Read the model definition and answer for the solid it produces. Units are mm, in the model's axes. A direction names the side the tool comes from. Give positions to 0.01 mm unless a question says otherwise; leave off trailing zeros. Write each loop counter-clockwise with the first axis right and the second up, starting at its lowest first coordinate (ties: lowest second). Pieces come first, ordered by that corner, then holes. Notation, with made-up numbers: M -14,43 L 45,43 A19 ccw 45,48 Z; hole C 12.5,14.5 d8. An arc over 180 degrees is marked long. Put each result on its own line as item: value.
from build123d import *

# Parameters (mm, degrees)
SKETCH1_R           = 12.7
EXTRUDE1_DEPTH      = 11.1125
EXTRUDE2_DEPTH      = 23.225
SKETCH4_R           = 2.3876
BOSS_EXTRUDE1_DEPTH = 19.05


with BuildPart() as part:
    # Sketch1 → Extrude1 (new body, symmetric)
    with BuildSketch(Plane.XY):
        Circle(SKETCH1_R)
    extrude(amount=EXTRUDE1_DEPTH, both=True)

    # Sketch2 → Extrude2 (cut, through all)
    with BuildSketch(Plane.XY.offset(11.1125)):
        with BuildLine():
            ThreePointArc((0.79375, 2.24506403), (0, 2.38125), (-0.79375, 2.24506403))
            Line((-0.79375, 2.24506403), (-0.79375, 1.5875))
            Line((-0.79375, 1.5875), (0.79375, 1.5875))
            Line((0.79375, 1.5875), (0.79375, 2.24506403))
        make_face()
        with BuildLine():
            Line((-0.79375, 1.5875), (-0.79375, 2.24506403))
            ThreePointArc((-0.79375, 2.24506403), (-1.374815329, -1.944282483), (2.38125, 0))
            ThreePointArc((2.38125, 0), (1.944282483, 1.374815329), (0.79375, 2.24506403))
            Line((0.79375, 2.24506403), (0.79375, 1.5875))
            Line((0.79375, 1.5875), (-0.79375, 1.5875))
        make_face()
        with BuildLine():
            Line((0.79375, 3.175), (-0.79375, 3.175))
            Line((-0.79375, 3.175), (-0.79375, 2.24506403))
            ThreePointArc((-0.79375, 2.24506403), (0, 2.38125), (0.79375, 2.24506403))
            Line((0.79375, 2.24506403), (0.79375, 3.175))
        make_face()
    extrude(amount=-EXTRUDE2_DEPTH, mode=Mode.SUBTRACT)

    # Sketch4 → Boss-Extrude1 (add, symmetric)
    with BuildSketch(Plane.XY):
        Circle(SKETCH4_R)
    extrude(amount=BOSS_EXTRUDE1_DEPTH, both=True)


solid = part.part
(1) Section B-B on z = -1 is taken. Determine the outline of the cut face in (x, y) (3 decimals).
Result:
outline: C 0,0 d25.4; hole M -0.794,2.252 A2.388 cw 0.794,2.252 L 0.794,3.175 L -0.794,3.175 Z
(2) Straight lines are drawn through the part: line 1 along Z through (x, y) = (-1.25, -9); line 2 along Y through (x, z) = (-0.5, 2) (3 decimals); line 3 along X through (y, z) = (-9.75, -5). For each, find the intervals that lie inside material, in ascending order. Write a range as from..to.
Result:
line 1: z = -11.11..11.11
line 2: y = -12.69..2.335, 3.175..12.69
line 3: x = -8.14..8.14
(3) For a pull along Y with two mould halves and no side action, classify faces 4 (the face through (0, -3, -11.112)), 5 (the face through (0.794, 3, 0)), 6 (the face through (-2.75, -12.4, 0.16)) as +Y half, -Y half, draft (parallel to the pull), parting line (faces both ways), or undercut.
Result:
face 4: draft
face 5: undercut
face 6: parting line
(4) Section C-C on y = 0 is taken. Determine the outline of the cut face in (x, z), and give its area (3 significant figures).
Result:
outline: M -12.7,-11.11 L -2.39,-11.11 L -2.39,-19.05 L 2.39,-19.05 L 2.39,-11.11 L 12.7,-11.11 L 12.7,11.11 L 2.39,11.11 L 2.39,19.05 L -2.39,19.05 L -2.39,11.11 L -12.7,11.11 Z
area: 640 mm²
(5) Given pin 1 Ø8 at (y, z) = (-7, 1) entering from +X; pin 2 Ø1 at (x, z) = (8.5, -0.5) entering from +Y; pin 3 Ø10 at (y, z) = (9.5, 4.5) entering from +X; pin 4 Ø12.5 at (x, y) = (-2.5, -1.5) entering from -Z, each flat-ended and moving along its own axis, determine where each tip first touches the part or whether it passes through.
Result:
pin 1: stops at x = 12.34
pin 2: stops at y = 9.86
pin 3: stops at x = 11.88
pin 4: stops at z = -19.05
(6) Which of the six approach directions +Z, -Z, +X, -X, +Y, -Y give full straight-line access (tool end or side, diameter ignored) to faces 1 (the face through (0, 0, 19.05)), 2 (the face through (-0.311, 2.367, 0.267)), 3 (the face through (0, 3.175, 0))?
Result:
face 1: +Z, +X, -X, +Y, -Y
face 2: none
face 3: +Z, -Z
(7) Section D-D on z = -13 is taken. Determine the outline of the cut face in (x, y), and give its area (3 significant figures).
Result:
outline: C 0,0 d4.78
area: 17.9 mm²
